```python
from build123d import *

# Parameters (mm, degrees)
CUT_EXTRUDE_1_DEPTH      = 65
CUT_EXTRUDE_1_DEPTH_BACK = 65
CUT_EXTRUDE_2_DEPTH      = 65
CUT_EXTRUDE_2_DEPTH_BACK = 65
CUT_EXTRUDE_3_DEPTH      = 65
CUT_EXTRUDE_3_DEPTH_BACK = 65
CUT_EXTRUDE_4_DEPTH      = 65
CUT_EXTRUDE_4_DEPTH_BACK = 65


with BuildPart() as part:
    # Sketch 1 → Revolve 1 (revolve)
    with BuildSketch(Plane(origin=(0, 0, 0), x_dir=(0, 0, -1), z_dir=(1, 0, 0)), mode=Mode.PRIVATE) as revolve_1_sk:
        Polygon((0, 46), (0, 65), (56, 65), (56, 46), (126, 46), (126, 32), (123, 32), (123, 34), (45, 34), (45, 46), align=None)
    revolve(revolve_1_sk.sketch.rotate(Axis((0, 0, 0), (0, 0, -1)), 90), axis=Axis((0, 0, 0), (0, 0, -1)))

    # Sketch 2 → Cut-Extrude 1 (cut, two sides: drawn at the far end of the back side and taken through both)
    with BuildSketch(Plane(origin=(0, 0, 0), x_dir=(0, 0, -1), z_dir=(1, 0, 0)).offset(-CUT_EXTRUDE_1_DEPTH_BACK)):
        Polygon((0, 16), (0, -16), (32, -8), (32, 8), align=None)
    extrude(amount=CUT_EXTRUDE_1_DEPTH + CUT_EXTRUDE_1_DEPTH_BACK, mode=Mode.SUBTRACT)

    # Sketch 3 → Cut-Extrude 2 (cut, two sides: drawn at the far end of the back side and taken through both)
    with BuildSketch(Plane(origin=(0, 0, 0), x_dir=(1, 0, 0), z_dir=(0, 1, 0)).offset(-CUT_EXTRUDE_2_DEPTH_BACK)):
        Polygon((-16, 0), (16, 0), (8, 32), (-8, 32), align=None)
    extrude(amount=CUT_EXTRUDE_2_DEPTH + CUT_EXTRUDE_2_DEPTH_BACK, mode=Mode.SUBTRACT)

    # Sketch 4 → Cut-Extrude 3 (cut, two sides: drawn at the far end of the back side and taken through both)
    with BuildSketch(Plane(origin=(0, 0, 0), x_dir=(-0.7071067811865476, -0.7071067811865475, 0), z_dir=(-0.7071067811865475, 0.7071067811865476, 0)).offset(-CUT_EXTRUDE_3_DEPTH_BACK)):
        Polygon((16, 0), (-16, 0), (-8, -32), (8, -32), align=None)
    extrude(amount=CUT_EXTRUDE_3_DEPTH + CUT_EXTRUDE_3_DEPTH_BACK, mode=Mode.SUBTRACT)

    # Sketch 5 → Cut-Extrude 4 (cut, two sides: drawn at the far end of the back side and taken through both)
    with BuildSketch(Plane(origin=(0, 0, 0), x_dir=(0, 0, -1), z_dir=(0.7071067811865476, 0.7071067811865475, 0)).offset(-CUT_EXTRUDE_4_DEPTH_BACK)):
        Polygon((0, 16), (0, -16), (32, -8), (32, 8), align=None)
    extrude(amount=CUT_EXTRUDE_4_DEPTH + CUT_EXTRUDE_4_DEPTH_BACK, mode=Mode.SUBTRACT)


solid = part.part
```
Can you work these out from the model? Positions are in its coordinate system, mm. A direction names the side the tool comes from. Round coordinates to 2 decimals unless told otherwise and drop trailing zeros. Order: outer loops, then holes, each group sorted by start corner. A loop starts at its lowest first (then second) coordinate and runs counter-clockwise, first axis right, second up. Notation, with made-up numbers: (66, 74) -> (109, 74) arc R26 cw to (109, 108) -> close; hole circle Ø1 at (64.5, 58.25). An arc over 180 degrees is marked (long way). Return JSON: item names as keys, results as strings. Group by question number.
1. I need wall thicknesses on line 1 (Y direction, x = 0, z = -77); line 2 (Z direction, x = 5.5, y = -53); line 3 (Z direction, x = 3, y = 40). Which ranges of each line are inside material? Lowest first, please. Write a range as [from, to].
2. Will these pins go through, and if not, where does the flat tip stop? pin 1 (10 mm diameter, centred on y = -20, z = -49.5, fed in from +X); pin 2 (1.5 mm diameter, centred on y = -2.5, z = -91.5, fed in from -X); pin 3 (1 mm diameter, centred on x = -2.5, y = 37.5, fed in from +Z); pin 4 (20.5 mm diameter, centred on x = 16.5, y = 13, fed in from +Z).
3. Which directions (+Z, -Z, +X, -X, +Y, -Y) give clear straight access to the entire face, cutting with the end or side of a thin tool? Please do faces 1 (the face through (54, -12, -16)), 2 (the face through (39, 39, -32)), 3 (the face through (0, -55, -32)).
4. We'd pull the mould along Y, two halves only. Please class faces 4 (the face through (-5.99, -45.61, -91.49)), 5 (the face through (39, -39, -32)), 6 (the face through (23, -53, 0)): released by +Y, released by -Y, zero draft, split by the parting line, or undercut.
5. If we section it at D-D, the plane z = -75.5: Write out the boundary of the cut face in (x, y), then the cut area to 3 significant figures.
6. If we section it at A-A, the plane x = 0: Write out the boundary of the cut face in (y, z), then the cut area to 3 significant figures.
7. If we section it at C-C, the plane z = -27.5: Count the separate pieces of the cut face and the enclosed holes in it, then the cut area to 3 significant figures.
Output values:
{
 "1": {"line 1": "[-46, -34], [34, 46]", "line 2": "[-56, -32]", "line 3": "[-126, -45]"},
 "2": {"pin 1": "x = 63.25", "pin 2": "x = -45.97", "pin 3": "z = -45", "pin 4": "through"},
 "3": {"face 1": "+Z, +X, -X", "face 2": "+Z", "face 3": "+Z, +Y, -Y"},
 "4": {"face 4": "split by the parting line", "face 5": "undercut", "face 6": "zero draft"},
 "5": {"outline": "circle Ø92 at (0, 0); hole circle Ø68 at (0, 0)", "area": "3,020 mm²"},
 "6": {"outline": "(-65, -56) -> (-46, -56) -> (-46, -126) -> (-32, -126) -> (-32, -123) -> (-34, -123) -> (-34, -45) -> (-46, -45) -> (-46, -32) -> (-65, -32) -> close; (32, -126) -> (46, -126) -> (46, -56) -> (65, -56) -> (65, -32) -> (46, -32) -> (46, -45) -> (34, -45) -> (34, -123) -> (32, -123) -> close", "area": "2,870 mm²"},
 "7": {"separate pieces": "8", "enclosed holes": "0", "area": "3,840 mm²"}
}
